from build123d import *

# Parameters (mm, degrees)
ESQUISSE1_R                  = 57.75
ESQUISSE1_R_2                = 4
BOSS_EXTRU_1_DEPTH           = 1
ENL_V_MAT_EXTRU_1_DEPTH      = 82.676955134
ENL_V_MAT_EXTRU_1_DEPTH_BACK = 82.676955134
ESQUISSE2_R                  = 1.53
ENL_V_MAT_EXTRU_2_DEPTH      = 1


with BuildPart() as part:
    # Esquisse1 → Boss.-Extru.1 (new body)
    with BuildSketch(Plane.XY):
        Circle(ESQUISSE1_R)
        Circle(ESQUISSE1_R_2, mode=Mode.SUBTRACT)
    extrude(amount=BOSS_EXTRU_1_DEPTH)

    # Esquisse2 → Enlèv. mat.-Extru.1 (cut, two sides: drawn at the far end of the back side and taken through both)
    with BuildSketch(Plane(origin=(0, 0, 0), x_dir=(-1, 0, 0), z_dir=(0, 0, -1)).offset(-ENL_V_MAT_EXTRU_1_DEPTH_BACK)):
        with Locations((0, -15.504004846)):
            Circle(ESQUISSE2_R)
    extrude(amount=ENL_V_MAT_EXTRU_1_DEPTH + ENL_V_MAT_EXTRU_1_DEPTH_BACK, mode=Mode.SUBTRACT)

    # Esquisse3 → Enlèv. mat.-Extru.2 (cut)
    with BuildSketch(Plane(origin=(0, 0, 0), x_dir=(-1, 0, 0), z_dir=(0, 0, -1))):
        with BuildLine():
            Line((19.755068189, -28.89182031), (32.389647952, -46.281827468))
            ThreePointArc((32.389647952, -46.281827468), (25.70214401, -50.443439565), (18.405179994, -53.409251489))
            Line((18.405179994, -53.409251489), (11.76223589, -32.96437178))
            ThreePointArc((11.76223589, -32.96437178), (15.889667491, -31.185228347), (19.755068189, -28.89182031))
        make_face()
    extrude(amount=-ENL_V_MAT_EXTRU_2_DEPTH, mode=Mode.SUBTRACT)


solid = part.part
Design review of the part built by this model. Coordinates are the model's own, in mm. A direction names the side the tool comes from. Coordinates: 2 decimals unless noted, no trailing zeros. Order: outer loops, then holes, each group sorted by start corner. A loop starts at its lowest first (then second) coordinate and runs counter-clockwise, first axis right, second up. Notation, with made-up numbers: M 87.25,53 L 117.25,53 A18 cw 117.25,79 Z; hole C 34,-15 d7. An arc over 180 degrees is marked long. Use a Markdown table: item, result.
(1) Add section A-A (y = 0). Give the boundary of the cut face in (x, z).
Worked answers:
| item | result |
|---|---|
| outline | M -57.75,0 L -4,0 L -4,1 L -57.75,1 Z; M 4,0 L 57.75,0 L 57.75,1 L 4,1 Z |
(2) For faces 4 (the flat face through (12, 1, 1)), 5 (the flat face through (-25.984, -37.465, 0.493)), list the 3-axis set-ups (+Z, -Z, +X, -X, +Y, -Y) from which the entire face can be reached by the end or side of a thin tool; tool diameter is ignored.
Worked answers:
| item | result |
|---|---|
| face 4 | +Z, +X, -X, +Y, -Y |
| face 5 | +Z, -Z |
(3) For P1, Ø5, axis at x = 0, y = -15.5, coming from the +Z side, flat-tipped, find the tip position at first contact; note if it passes through.
Worked answers:
| item | result |
|---|---|
| P1 | stops at z = 1 |
(4) Wall thickness on probe 1 along Y at (x, z) = (0, 0.55); probe 2 along Y at (x, z) = (-3.5, 0.15); probe 3 along X at (y, z) = (2, 0.95): over which ranges is each line inside the solid? List them lowest first.
Worked answers:
| item | result |
|---|---|
| probe 1 | y = -57.75 to -17.03, -13.97 to -4, 4 to 57.75 |
| probe 2 | y = -57.64 to -1.94, 1.94 to 57.64 |
| probe 3 | x = -57.72 to -3.46, 3.46 to 57.72 |
(5) Add section B-B (x = 0). Give the boundary of the cut face in (y, z), then the cut area to 3 significant figures.
Worked answers:
| item | result |
|---|---|
| outline | M -57.75,0 L -17.03,0 L -17.03,1 L -57.75,1 Z; M -13.97,0 L -4,0 L -4,1 L -13.97,1 Z; M 4,0 L 57.75,0 L 57.75,1 L 4,1 Z |
| area | 104 mm2 |
(6) Draft analysis for pull direction X (two halves, no side actions). For faces 1 (the flat face through (12, 1, 0)), 2 (the cylindrical face through (-45.83, -35.14, 0.49)), 3 (the cylindrical face through (-25.8, -50.393, 0.493)), state which applies: released by +X, released by -X, zero draft, split by the parting line, or undercut.
Worked answers:
| item | result |
|---|---|
| face 1 | zero draft |
| face 2 | split by the parting line |
| face 3 | undercut |
(7) Add section D-D (x = -13.5). Give the boundary of the cut face in (y, z).
Worked answers:
| item | result |
|---|---|
| outline | M -56.15,0 L -38.31,0 L -38.31,1 L -56.15,1 Z; M -32.29,0 L 56.15,0 L 56.15,1 L -32.29,1 Z |
(8) Add section C-C (z = 0.85). Give the boundary of the cut face in (x, y), then the cut area to 3 significant figures.
Worked answers:
| item | result |
|---|---|
| outline | C 0,0 d115.5; hole M -32.39,-46.28 A46.23 ccw -18.41,-53.41 L -11.76,-32.96 A35 cw -19.76,-28.89 Z; hole C 0,0 d8; hole C 0,-15.5 d3.06 |
| area | 10,200 mm2 |
